For this review, take the finished solid that the model builds, in its own axes (mm). A direction names the side the tool comes from. Give positions to 0.01 mm unless a question says otherwise; leave off trailing zeros. Loops run counter-clockwise (first coordinate to the right, second up) from the corner with the lowest first, then second, coordinate; pieces in that order, holes last. Notation, with made-up numbers: (88, 47) - (140, 47) arc R21 ccw to (140, 65) - close; hole circle Ø5 at (38.25, -17). An arc over 180 degrees is marked (long way). Use CSV: the item, a comma, the result in double quotes. Start each with the question number.
1. Take a section at A-A on z = -494.5. Give the boundary of the cut face in (x, y).
2. For faces 5 (the flat face through (-906, 433, -283.16)), 6 (the flat face through (-343.255, 433, -500)), 7 (the flat face through (-905, 433, -393.164)), 8 (the flat face through (-122.617, 200, -399)), list the 3-axis set-ups (+Z, -Z, +X, -X, +Y, -Y) from which the entire face can be reached by the end or side of a thin tool; tool diameter is ignored.
3. Take a section at B-B on y = 151.5. Give the boundary of the cut face in (x, z) (1 decimal).
4. Mouldability with a two-part tool opening along X and no side actions: class faces 1 (the flat face through (-613, 482.6, -680)), 2 (the flat face through (-489.927, 433, -342)), 3 (the flat face through (-730, 171, -689.172)), 4 (the flat face through (-430.851, 433, -501)) as pulls with the +X half, pulls with the -X half, needs draft (parallel to the pull), parting line crosses it, or undercut.
5. Take a section at D-D on y = 433.5. Give the boundary of the cut face in (x, z).
6. For pin 1 (4 mm diameter, centred on x = -367, y = 174, fed in from +Z); pin 2 (5 mm diameter, centred on y = 153.5, z = -397, fed in from +X); pin 3 (10 mm diameter, centred on y = 413.5, z = -370, fed in from +X), all flat-tipped, find the tip position at first contact; note any pin that passes through.
7. Wall thickness on line 1 (Z direction, x = -382.5, y = 447.5); line 2 (Y direction, x = -206, z = -631); line 3 (Z direction, x = -475.5, y = 246.5): over which ranges is each line inside the solid? List them lowest first.
8. Take a section at C-C on x = -415. Give the boundary of the cut face in (y, z).
Autodesk Inventor part; units mm, degrees
ref_plane "YZ Plane" through (0, 0, 0) normal (1, 0, 0) x (0, 1, 0)
ref_plane "XZ Plane" through (0, 0, 0) normal (0, 1, 0) x (-1, 0, 0)
ref_plane "XY Plane" through (0, 0, 0) normal (0, 0, 1) x (1, 0, 0)
sketch "Sketch1" plane through (0, 0, 0) normal (0, 1, 0) x (-1, 0, 0)
  line L0 (0, 0) -> (1219.2, 0)
  line L1 (1219.2, 0) -> (1219.2, -1219.2)
  line L2 (1219.2, -1219.2) -> (0, -1219.2)
  line L3 (0, -1219.2) -> (0, 0)
  dimension "d0" = 1219.2
  dimension "d1" = 1219.2
extrude "Extrusion1" add sketch "Sketch1" along normal blind 25.4
sketch "Sketch2" plane through (0, 25.4, 0) normal (0, 1, 0) x (1, 0, 0)
  line L0 (-1088.9403, 92.3181) -> (-122.6171, 92.3181)
  line L1 (-122.6171, 92.3181) -> (-122.6171, 714.5717)
  line L2 (-122.6171, 714.5717) -> (-1088.9403, 714.5717)
  line L3 (-1088.9403, 714.5717) -> (-1088.9403, 92.3181)
  point P0 (0, 0)
extrude "Extrusion2" add sketch "Sketch2" along normal blind 457.2
sketch "Sketch3" plane through (0, 482.6, 0) normal (0, 1, 0) x (1, 0, 0)
  line L0 (-1088.9403, 92.3181) -> (-1088.9403, 714.5717)
  line L1 (-122.6171, 92.3181) -> (-122.6171, 714.5717)
  line L2 (-1088.9403, 643.7299) -> (-122.6171, 643.7299)
  line L3 (-122.6171, 643.7299) -> (-122.6171, 92.3181)
  line L4 (-122.6171, 92.3181) -> (-1088.9403, 92.3181)
  line L5 (-1088.9403, 92.3181) -> (-1088.9403, 643.7299)
  line L6 (-954.3907, 283.1597) -> (-856.609, 283.1597)
  line L7 (-856.609, 283.1597) -> (-856.609, 393.1642)
  line L8 (-856.609, 393.1642) -> (-954.3907, 393.1642)
  line L9 (-954.3907, 393.1642) -> (-954.3907, 283.1597)
  line L10 (-430.8509, 462.4262) -> (-343.2547, 462.4262)
  line L11 (-343.2547, 462.4262) -> (-343.2547, 537.7997)
  line L12 (-343.2547, 537.7997) -> (-430.8509, 537.7997)
  line L13 (-430.8509, 537.7997) -> (-430.8509, 462.4262)
  circle A0 centre (-791.4211, 232.2317) radius 53.9356
  circle A1 centre (-650.8599, 232.2317) radius 56.421
  line L14 (-489.9274, 288.6527) -> (-387.0528, 288.6527)
  line L15 (-387.0528, 288.6527) -> (-387.0528, 393.1642)
  line L16 (-387.0528, 393.1642) -> (-489.9274, 393.1642)
  line L17 (-489.9274, 393.1642) -> (-489.9274, 288.6527)
  point P0 (0, 0)
extrude "Extrusion3" cut sketch "Sketch3" against normal blind 101.6
sketch "Sketch4" plane through (-122.6171, 25.4, -714.5717) normal (0, 0, -1) x (-1, 0, 0)
  line L0 (0, 0) -> (966.3232, 0)
  line L1 (243.2512, 0) -> (327.8074, 0)
  line L2 (327.8074, 0) -> (327.8074, 181.9254)
  line L3 (327.8074, 181.9254) -> (243.2512, 181.9254)
  line L4 (243.2512, 181.9254) -> (243.2512, 0)
  line L5 (456.2679, 216.0731) -> (763.5973, 216.0731)
  line L6 (763.5973, 216.0731) -> (763.5973, 72.9779)
  line L7 (763.5973, 72.9779) -> (456.2679, 72.9779)
  line L8 (456.2679, 72.9779) -> (456.2679, 216.0731)
  line L9 (26.9824, 216.0731) -> (196.0948, 216.0731)
  line L10 (196.0948, 216.0731) -> (196.0948, 72.9779)
  line L11 (196.0948, 72.9779) -> (26.9824, 72.9779)
  line L12 (26.9824, 72.9779) -> (26.9824, 216.0731)
  point P0 (-122.6171, -25.4)
extrude "Extrusion4" cut sketch "Sketch4" against normal blind 25.4
equation "\"d1\" = d0"
properties part number "building_1" material "Wood (Oak)"
Check result:
1,outline,"(-1219.2, 0) - (0, 0) - (0, 25.4) - (-122.62, 25.4) - (-122.62, 381) - (-343.25, 381) - (-343.25, 482.6) - (-430.85, 482.6) - (-430.85, 381) - (-1088.94, 381) - (-1088.94, 25.4) - (-1219.2, 25.4) - close"
2,face 5,"+Z, -X, +Y"
2,face 6,"+Z, +X, +Y"
2,face 7,"+X, -X, +Y"
2,face 8,"+Z, -Z, +X, +Y"
3,outline,"(-1088.9, -714.6) - (-886.2, -714.6) - (-886.2, -689.2) - (-578.9, -689.2) - (-578.9, -714.6) - (-450.4, -714.6) - (-450.4, -689.2) - (-365.9, -689.2) - (-365.9, -714.6) - (-318.7, -714.6) - (-318.7, -689.2) - (-149.6, -689.2) - (-149.6, -714.6) - (-122.6, -714.6) - (-122.6, -92.3) - (-1088.9, -92.3) - close"
4,face 1,"needs draft"
4,face 2,"undercut"
4,face 3,"undercut"
4,face 4,"pulls with the -X half"
5,outline,"(-1088.94, -714.57) - (-122.62, -714.57) - (-122.62, -643.73) - (-1088.94, -643.73) - close; (-954.39, -393.16) - (-856.61, -393.16) - (-856.61, -283.16) - (-954.39, -283.16) - close; circle Ø107.87 at (-791.42, -232.23); circle Ø112.84 at (-650.86, -232.23); (-489.93, -393.16) - (-387.05, -393.16) - (-387.05, -288.65) - (-489.93, -288.65) - close; (-430.85, -537.8) - (-343.25, -537.8) - (-343.25, -462.43) - (-430.85, -462.43) - close"
6,pin 1,"stops at z = -92.32"
6,pin 2,"stops at x = -122.62"
6,pin 3,"stops at x = -387.05"
7,line 1,"z = -714.57 to -643.73, -537.8 to -462.43"
7,line 2,"y = 0 to 381"
7,line 3,"z = -714.57 to -92.32"
8,outline,"(0, -1219.2) - (25.4, -1219.2) - (25.4, -689.17) - (207.33, -689.17) - (207.33, -714.57) - (482.6, -714.57) - (482.6, -643.73) - (381, -643.73) - (381, -537.8) - (482.6, -537.8) - (482.6, -462.43) - (381, -462.43) - (381, -393.16) - (482.6, -393.16) - (482.6, -288.65) - (381, -288.65) - (381, -92.32) - (25.4, -92.32) - (25.4, 0) - (0, 0) - close"
